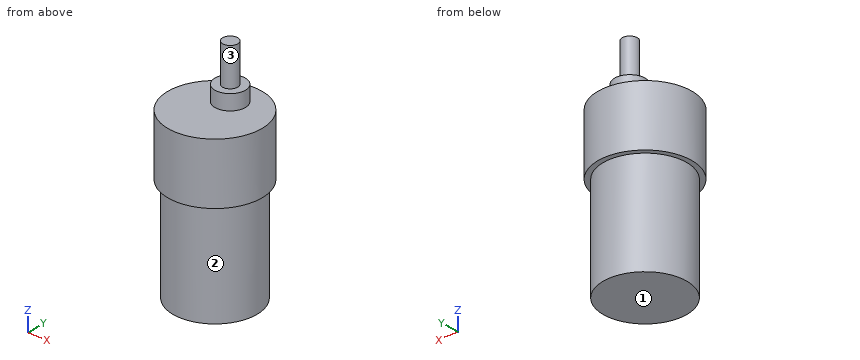
from build123d import *

# Parameters (mm, degrees)
SKETCH1_R           = 16.5
BOSS_EXTRUDE1_DEPTH = 20.5
SKETCH2_R           = 18.5
BOSS_EXTRUDE2_DEPTH = 24
SKETCH3_R           = 6
BOSS_EXTRUDE3_DEPTH = 6
SKETCH4_R           = 3
BOSS_EXTRUDE4_DEPTH = 15


with BuildPart() as part:
    # Sketch1 → Boss-Extrude1 (new body, symmetric)
    with BuildSketch(Plane.XY):
        Circle(SKETCH1_R)
    extrude(amount=BOSS_EXTRUDE1_DEPTH, both=True)

    # Sketch2 → Boss-Extrude2 (add)
    with BuildSketch(Plane.XY.offset(20.5)):
        Circle(SKETCH2_R)
    extrude(amount=BOSS_EXTRUDE2_DEPTH)

    # Sketch3 → Boss-Extrude3 (add)
    with BuildSketch(Plane.XY.offset(44.5)):
        with Locations((0, 7)):
            Circle(SKETCH3_R)
    extrude(amount=BOSS_EXTRUDE3_DEPTH)

    # Sketch4 → Boss-Extrude4 (add)
    with BuildSketch(Plane.XY.offset(50.5)):
        with Locations((0, 7)):
            Circle(SKETCH4_R)
    extrude(amount=BOSS_EXTRUDE4_DEPTH)


solid = part.part
CAD build for the part. Positions are in the model's coordinates, mm. Face numbers are marked on the shaded views. A direction names the side the tool comes from. Round coordinates to 2 decimals unless told otherwise and drop trailing zeros. Loops run counter-clockwise (first coordinate to the right, second up) from the corner with the lowest first, then second, coordinate; pieces in that order, holes last. Notation, with made-up numbers: (58.25, 59) - (90.25, 59) arc R20 ccw to (90.25, 94) - close; hole circle Ø10 at (48, 6). An arc over 180 degrees is marked (long way). Put each result on its own line as item: value.
1. Slice it at A-A on x = 0. List the corners of the cut face in (y, z).
Geometry check:
outline: (-18.5, 20.5) - (-16.5, 20.5) - (-16.5, -20.5) - (16.5, -20.5) - (16.5, 20.5) - (18.5, 20.5) - (18.5, 44.5) - (13, 44.5) - (13, 50.5) - (10, 50.5) - (10, 65.5) - (4, 65.5) - (4, 50.5) - (1, 50.5) - (1, 44.5) - (-18.5, 44.5) - close
2. Wall check: line 1 (Z direction, x = 11, y = 1.5); line 2 (Z direction, x = -5, y = 5); line 3 (X direction, y = 2.5, z = 0.5). Give the ranges that are in metal, low to high.
Geometry check:
line 1: -20.5 to 44.5
line 2: -20.5 to 50.5
line 3: -16.31 to 16.31
3. Slice it at D-D on x = -13.5. List the corners of the cut face in (y, z), and give its area (3 significant figures).
Geometry check:
outline: (-12.65, 20.5) - (-9.49, 20.5) - (-9.49, -20.5) - (9.49, -20.5) - (9.49, 20.5) - (12.65, 20.5) - (12.65, 44.5) - (-12.65, 44.5) - close
area: 1,390 mm²
4. Pin check, flat tips, straight feed: P1, Ø1, axis at x = 11, y = -9, coming from the +Z side; P2, Ø5, axis at y = -8.5, z = 49, coming from the +X side; P3, Ø10, axis at x = 0.5, z = 34, coming from the +Y side; P4, Ø12, axis at x = 10, z = 2, coming from the -Y side. Stop position of each tip, or through.
Geometry check:
P1: z = 44.5
P2: through
P3: y = 18.5
P4: y = -16.01
5. Slice it at B-B on y = 0. List the corners of the cut face in (x, z).
Geometry check:
outline: (-18.5, 20.5) - (-16.5, 20.5) - (-16.5, -20.5) - (16.5, -20.5) - (16.5, 20.5) - (18.5, 20.5) - (18.5, 44.5) - (-18.5, 44.5) - close
6. Slice it at C-C on z = -4.5. List the corners of the cut face in (x, y), and give its area (3 significant figures).
Geometry check:
outline: circle Ø33 at (0, 0)
area: 855 mm²
7. 3-axis set-ups, long thin cutter, end or side, ignore diameter. For the marked faces 1, 2 and 3: which of +Z, -Z, +X, -X, +Y, -Y reach the whole face in a straight line?
Geometry check:
face 1: -Z, +X, -X, +Y, -Y
face 2: -Z
face 3: +Z
